Part model, mm, in its own coordinate system. Face numbers are marked on the shaded views. A direction names the side the tool comes from. Round coordinates to 2 decimals unless told otherwise and drop trailing zeros. Write each loop counter-clockwise with the first axis right and the second up, starting at its lowest first coordinate (ties: lowest second). Pieces come first, ordered by that corner, then holes. Notation, with made-up numbers: M 47,-20.5 L 80,-20.5 A32 cw 80,15.5 Z; hole C 25.5,-10.75 d10. An arc over 180 degrees is marked long. Answer as a JSON object with one key per item and string values. Group by question number.
1. Two-plate mould, pull along Z, no slides. Class the marked faces 1, 2, 3 and 4: +Z half, -Z half, draft (parallel to the pull), parting line (faces both ways), or undercut.
2. Drop flat-ended pins along their axis: pin 1 (3 mm diameter, centred on x = 5, y = 51.5, fed in from -Z); pin 2 (8 mm diameter, centred on y = 43, z = -6.5, fed in from -X); pin 3 (3 mm diameter, centred on x = 5.5, y = 24, fed in from +Z); pin 4 (3 mm diameter, centred on x = 5.5, z = -4, fed in from +Y). Give the stop position or say it passes through.
3. Drill centre lines: line 1 (Y direction, x = 5, z = 14.4); line 2 (Z direction, x = 2.25, y = 55.5); line 3 (X direction, y = 1.35, z = -6). Where is each one in solid material? Low to high. Write a range as from..to.
4. Band-saw the part on C-C, the plane x = 1.5. Write the cut outline in (y, z).
5. Band-saw the part on D-D, the plane z = 15. Write the cut outline in (x, y).
6. Band-saw the part on B-B, the plane z = -6. Write the cut outline in (x, y).
7. Which spindle directions (+Z, -Z, +X, -X, +Y, -Y) get a long thin tool onto all of the face, cutting with end or side? Do the marked faces 5, 6, 7 and 8. Say none if no direction does.
8. Band-saw the part on A-A, the plane y = 56. Write the cut outline in (x, z), plus the area to 3 significant figures.
from build123d import *

# Parameters (mm, degrees)
IZIM1_W                          = 10
IZIM1_H                          = 60
Y_KSEKLIK_EKSTR_ZYON1_DEPTH      = 16
Y_KSEKLIK_EKSTR_ZYON2_DEPTH      = 12
Y_KSEKLIK_EKSTR_ZYON2_DEPTH_BACK = 28
IZIM2_W                          = 10
IZIM2_H                          = 5
IZIM3_W                          = 9
IZIM3_H                          = 16
KES_EKSTR_ZYON2_DEPTH            = 12
IZIM4_R                          = 1.7
KES_EKSTR_ZYON3_DEPTH            = 25
IZIM5_R                          = 1.7
KES_EKSTR_ZYON4_DEPTH            = 25


with BuildPart() as part:
    # Çizim1 → Yükseklik-Ekstrüzyon1 (new body)
    with BuildSketch(Plane.XY):
        with Locations((5, 30)):
            Rectangle(IZIM1_W, IZIM1_H)
    extrude(amount=Y_KSEKLIK_EKSTR_ZYON1_DEPTH)

    # Çizim2 → Yükseklik-Ekstrüzyon2 (add, two sides: drawn at the far end of the back side and taken through both)
    with BuildSketch(Plane.XY.offset(16).offset(-Y_KSEKLIK_EKSTR_ZYON2_DEPTH_BACK)):
        with Locations((5, 2.5)):
            Rectangle(IZIM2_W, IZIM2_H)
    extrude(amount=Y_KSEKLIK_EKSTR_ZYON2_DEPTH + Y_KSEKLIK_EKSTR_ZYON2_DEPTH_BACK)

    # Çizim3 → Kes-Ekstrüzyon2 (cut)
    with BuildSketch(Plane(origin=(10, 0, 0), x_dir=(0, 0, -1), z_dir=(1, 0, 0))):
        with Locations((-8, 52)):
            Rectangle(IZIM3_W, IZIM3_H)
    extrude(amount=-KES_EKSTR_ZYON2_DEPTH, mode=Mode.SUBTRACT)

    # Çizim4 → Kes-Ekstrüzyon3 (cut)
    with BuildSketch(Plane.XY.offset(16)):
        with Locations((5, 56)):
            Circle(IZIM4_R)
    extrude(amount=-KES_EKSTR_ZYON3_DEPTH, mode=Mode.SUBTRACT)

    # Çizim5 → Kes-Ekstrüzyon4 (cut)
    with BuildSketch(Plane(origin=(0, 5, 0), x_dir=(1, 0, 0), z_dir=(0, 1, 0))):
        with Locations(Location((5, 6, 0), (0, 0, 270))):
            Circle(IZIM5_R)
        with Locations(Location((5, -22, 0), (0, 0, 270))):
            Circle(IZIM5_R)
    extrude(amount=-KES_EKSTR_ZYON4_DEPTH, mode=Mode.SUBTRACT)


solid = part.part
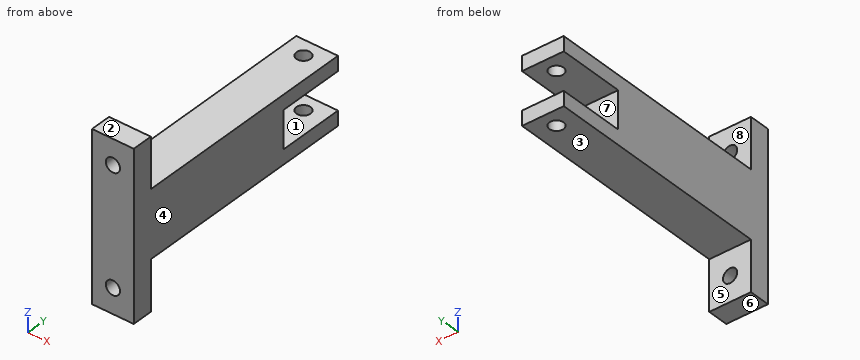
Worked answers:
{
 "1": {"face 1": "undercut", "face 2": "+Z half", "face 3": "-Z half", "face 4": "draft"},
 "2": {"pin 1": "stops at z = 0", "pin 2": "passes through", "pin 3": "stops at z = 16", "pin 4": "stops at y = 5"},
 "3": {"line 1": "y = 0..54.3, 57.7..60", "line 2": "z = 0..3.5, 12.5..16", "line 3": "x = 0..3.3, 6.7..10"},
 "4": {"outline": "M 0,-12 L 5,-12 L 5,0 L 60,0 L 60,3.5 L 44,3.5 L 44,12.5 L 60,12.5 L 60,16 L 5,16 L 5,28 L 0,28 Z"},
 "5": {"outline": "M 0,0 L 10,0 L 10,60 L 0,60 Z; hole C 5,56 d3.4"},
 "6": {"outline": "M 0,0 L 3.3,0 L 3.3,5 L 0,5 Z; M 6.7,0 L 10,0 L 10,5 L 6.7,5 Z"},
 "7": {"face 5": "-Z, +X, -X, +Y", "face 6": "-Z, +X, -X, +Y, -Y", "face 7": "+X, -X, +Y", "face 8": "+Z, +X, -X, +Y"},
 "8": {"outline": "M 0,0 L 3.3,0 L 3.3,3.5 L 0,3.5 Z; M 0,12.5 L 3.3,12.5 L 3.3,16 L 0,16 Z; M 6.7,0 L 10,0 L 10,3.5 L 6.7,3.5 Z; M 6.7,12.5 L 10,12.5 L 10,16 L 6.7,16 Z", "area": "46.2 mm^2"}
}
